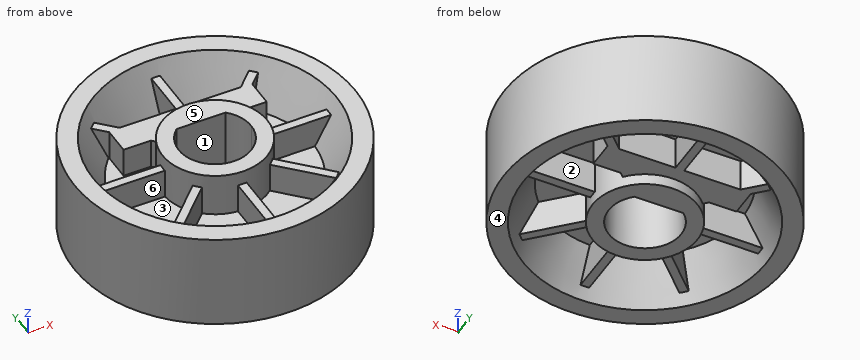
from build123d import *

# Parameters (mm, degrees)
SKETCH_2_R          = 5
CUT_EXTRUDE_1_DEPTH = 47.439853574
SKETCH_3_W          = 1.8
SKETCH_3_H          = 18
SKETCH_3_W_2        = 18
SKETCH_3_H_2        = 1.8
EXTRUDE_1_DEPTH     = 15
SKETCH_4_W          = 30
SKETCH_4_H          = 6
EXTRUDE_2_DEPTH     = 15
SCALE_1_SCALE       = 1.01


with BuildPart() as part:
    # Эскиз1 → Повернуть1 (revolve)
    with BuildSketch(Plane(origin=(0, 0, 0), x_dir=(1, 0, 0), z_dir=(0, 1, 0)), mode=Mode.PRIVATE) as revolve_1_sk:
        Polygon((-5, 0), (-11, 0), (-11, 9.3), (-20.5, 9.3), (-25.5, 0), (-29.5, 0), (-29.5, 20.4), (-25.5, 20.4), (-20.5, 11.1), (-11, 11.1), (-11, 20.4), (-5, 20.4), align=None)
    revolve(revolve_1_sk.sketch.rotate(Axis((0, 0, 0), (0, 0, -1)), 180), axis=Axis((0, 0, 0), (0, 0, -1)))

    # Эскиз2 → Вырез-Вытянуть1 (cut, through all)
    with BuildSketch(Plane.XY):
        with BuildLine():
            Line((5.138093031, 5.6), (-5.138093031, 5.6))
            ThreePointArc((-5.138093031, 5.6), (-3.058634741, -6.957352479), (7.6, 0))
            ThreePointArc((7.6, 0), (6.957352479, 3.058634741), (5.138093031, 5.6))
        make_face()
        Circle(SKETCH_2_R, mode=Mode.SUBTRACT)
    extrude(amount=-CUT_EXTRUDE_1_DEPTH, mode=Mode.SUBTRACT)

    # Эскиз3 → Бобышка-Вытянуть1 (add)
    with BuildSketch(Plane.XY.offset(-3)):
        Polygon((5.020458146, 6.293250353), (6.293250353, 5.020458146), (19.021172414, 17.748380208), (17.748380208, 19.021172414), align=None)
        with Locations((0, 17)):
            Rectangle(SKETCH_3_W, SKETCH_3_H)
        with Locations((17, 0)):
            Rectangle(SKETCH_3_W_2, SKETCH_3_H_2)
        Polygon((6.293250353, -5.020458146), (5.020458146, -6.293250353), (17.748380208, -19.021172414), (19.021172414, -17.748380208), align=None)
        with Locations((0, -17)):
            Rectangle(SKETCH_3_W, SKETCH_3_H)
        Polygon((-5.020458146, -6.293250353), (-6.293250353, -5.020458146), (-19.021172414, -17.748380208), (-17.748380208, -19.021172414), align=None)
        with Locations((-17, 0)):
            Rectangle(SKETCH_3_W_2, SKETCH_3_H_2)
        Polygon((-6.293250353, 5.020458146), (-5.020458146, 6.293250353), (-17.748380208, 19.021172414), (-19.021172414, 17.748380208), align=None)
    extrude(amount=-EXTRUDE_1_DEPTH)

    # Эскиз4 → Бобышка-Вытянуть2 (add)
    with BuildSketch(Plane.XY.offset(-3)):
        with Locations((0, 11)):
            Rectangle(SKETCH_4_W, SKETCH_4_H)
    extrude(amount=-EXTRUDE_2_DEPTH)


with BuildPart() as part_1:
    # Масштаб1: scaled about (0, 0.590334884, -10.24232435)
    add(part.part.scale(SCALE_1_SCALE).moved(Location((0, -0.005903349, 0.102423244))))


solid = part_1.part
For this review, take the finished solid that the model builds, in its own axes (mm). Face numbers are marked on the shaded views. A direction names the side the tool comes from. Round coordinates to 2 decimals unless told otherwise and drop trailing zeros. Loops run counter-clockwise (first coordinate to the right, second up) from the corner with the lowest first, then second, coordinate; pieces in that order, holes last. Notation, with made-up numbers: (35.5, 14.5) - (76.5, 14.5) arc R11 ccw to (76.5, 32.5) - close; hole circle Ø4 at (12.5, 6). An arc over 180 degrees is marked (long way). Use one line per item in the form item = value.
1) Wall thickness on probe 1 along X at (y, z) = (-1.5, -12.25); probe 2 along Y at (x, z) = (-12.5, -15); probe 3 along X at (y, z) = (19, -13.5): over which ranges is each line inside the solid? List them lowest first.
Solutions:
probe_1 = -29.76 to -21.27, -11.01 to -7.53, 7.53 to 11.01, 21.27 to 29.76
probe_2 = -27.05 to -19.07, -13.79 to -11.22, -0.91 to 0.9, 8.07 to 14.13, 19.06 to 27.04
probe_3 = -22.95 to -11.06, -0.91 to 0.91, 11.06 to 22.95
2) We need section A-A on x = 0. Write out the cut boundary in (y, z).
Solutions:
outline = (-29.8, -20.5) - (-25.76, -20.5) - (-24.46, -18.08) - (-11.12, -18.08) - (-11.12, -20.5) - (-7.68, -20.5) - (-7.68, 0.1) - (-11.12, 0.1) - (-11.12, -2.93) - (-24.13, -2.93) - (-25.76, 0.1) - (-29.8, 0.1) - close; (5.65, -20.5) - (11.1, -20.5) - (11.1, -18.08) - (24.45, -18.08) - (25.75, -20.5) - (29.79, -20.5) - (29.79, 0.1) - (25.75, 0.1) - (24.12, -2.93) - (11.1, -2.93) - (11.1, 0.1) - (5.65, 0.1) - close
3) Tool access review of the marked faces 1, 2, 3 and 4: name each direction out of +Z, -Z, +X, -X, +Y, -Y from which nothing blocks a thin tool from reaching the whole face with its end or side.
Solutions:
face_1 = +Z, -Z
face_2 = -Z
face_3 = +Z
face_4 = -Z, +X, -X, +Y, -Y
4) We need section B-B on z = -6. State how many separate pieces and enclosed holes the cut face has, then the cut area to 3 significant figures.
Solutions:
separate_pieces = 1
enclosed_holes = 9
area = 1,700 mm2
5) Clearance check with flat-ended pins moving along their axes: P1, Ø2, axis at x = -0.5, y = -18, coming from the -Z side; P2, Ø2, axis at x = 1, y = 23, coming from the +Z side; P3, Ø13.5, axis at x = 8, y = -16.5, coming from the +Z side. State where each tip first meets the part, or that it passes through.
Solutions:
P1 = -18.08
P2 = -2.93
P3 = -1.15
6) Mouldability with a two-part tool opening along Y and no side actions: class the marked faces 5 and 6 as pulls with the +Y half, pulls with the -Y half, needs draft (parallel to the pull), parting line crosses it, or undercut.
Solutions:
face_5 = needs draft
face_6 = undercut
